Source: CAD feature listing. Evaluate the final solid. Frame: model axes, mm. A direction names the side the tool comes from. Round coordinates to 2 decimals unless told otherwise and drop trailing zeros. Loops run counter-clockwise (first coordinate to the right, second up) from the corner with the lowest first, then second, coordinate; pieces in that order, holes last. Notation, with made-up numbers: (20, 27.5) - (71, 27.5) arc R21 cw to (71, 37.5) - close; hole circle Ø7 at (1.5, 81). An arc over 180 degrees is marked (long way). One line per question, with ' | ' between items. Start each with the question number.
1. Pin query (flat end, axial travel): pin 1 (3 mm diameter, centred on x = -3, y = -6, fed in from -Z); pin 2 (3.5 mm diameter, centred on x = -1.5, y = -7, fed in from +Z); pin 3 (2 mm diameter, centred on x = 22, z = 9.5, fed in from +Y); pin 4 (6 mm diameter, centred on y = -6.5, z = 9, fed in from +X). Return the tip coordinate at first contact, or that it passes through.
2. Mould query, pull axis X, two halves, no side actions, for faces 4 (the cylindrical face through (14.75, -4.11, 32.57)), 5 (the flat face through (13, -12, 16)), 6 (the flat face through (0, -6, 8)). Classes: pulls with the +X half, pulls with the -X half, needs draft (parallel to the pull), parting line crosses it, or undercut.
3. Access query for faces 1 (the flat face through (7.5, -6, 26)), 2 (the flat face through (8, -6, 31)), 3 (the flat face through (13, 0, 16)). Directions: +Z, -Z, +X, -X, +Y, -Y. A direction counts if a zero-diameter tool reaches every point of the face in a straight line with its end or side. Return the directions, or none.
4. Cut plane B-B (x = 25.5). Return loops of the section in (y, z), then the cut area to 3 significant figures.
5. Cut plane A-A (x = -3). Return loops of the section in (y, z).
6. Cut plane C-C (z = 19.5). Return loops of the section in (x, y) (1 decimal).
7. Ray query, line 1 (Y direction, x = -3, z = 20); line 2 (Y direction, x = 15, z = 32.3) (3 decimals); line 3 (Z direction, x = 23, y = -11). Return the intervals inside material, ascending.
8. Cut plane D-D (x = 15). Return loops of the section in (y, z) (3 decimals).
```python
from build123d import *

# Parameters (mm, degrees)
F0_W     = 10
F0_H     = 4
F0_W_2   = 15
F0_H_2   = 9
F1_DEPTH = 12
F2_R     = 1.5875
F3_DEPTH = 10
F4_R     = 6.35
F4_R_2   = 1.905
F5_DEPTH = 3.175


with BuildPart() as f1:
    # F0 (on Front) → F1 (new body)
    with BuildSketch(Plane.XZ):
        Polygon((0, 16), (0, 0), (22.5, 0), (22.5, 4), (22.5, 16), align=None)
        with Locations((27.5, 2)):
            Rectangle(F0_W, F0_H)
        Polygon((-5, 16), (0, 16), (22.5, 16), (27.5, 16), (27.5, 22), (22.5, 22), (7.5, 22), (-5, 22), align=None)
        with Locations((15, 26.5)):
            Rectangle(F0_W_2, F0_H_2)
    extrude(amount=F1_DEPTH)

    # F2 (on face) → F3 (cut)
    with BuildSketch(Plane.XY.offset(22)):
        with Locations((-3, -6)):
            Circle(F2_R)
        with Locations((25.5, -6)):
            Circle(F2_R)
    extrude(amount=-F3_DEPTH, mode=Mode.SUBTRACT)

    # F4 (on face) → F5 (join)
    with BuildSketch(Plane.XY.offset(31)):
        with Locations((15, -6)):
            Circle(F4_R)
        with Locations((15, -6)):
            Circle(F4_R_2, mode=Mode.SUBTRACT)
    extrude(amount=F5_DEPTH)


solid = f1.part
```
Answers follow:
1) pin 1: passes through | pin 2: stops at z = 22 | pin 3: stops at y = 0 | pin 4: stops at x = 22.5
2) face 4: undercut | face 5: needs draft | face 6: pulls with the -X half
3) face 1: +Z, -X, +Y, -Y | face 2: +Z, -X | face 3: -Z, +X, -X, +Y
4) outline: (-12, 0) - (0, 0) - (0, 4) - (-12, 4) - close; (-12, 16) - (-7.59, 16) - (-7.59, 22) - (-12, 22) - close; (-4.41, 16) - (0, 16) - (0, 22) - (-4.41, 22) - close | area: 101 mm2
5) outline: (-12, 16) - (-7.59, 16) - (-7.59, 22) - (-12, 22) - close; (-4.41, 16) - (0, 16) - (0, 22) - (-4.41, 22) - close
6) outline: (-5, -12) - (27.5, -12) - (27.5, 0) - (-5, 0) - close; hole circle Ø3.2 at (-3, -6); hole circle Ø3.2 at (25.5, -6)
7) line 1: y = -12 to -7.59, -4.41 to 0 | line 2: y = -12.35 to -7.905, -4.095 to 0.35 | line 3: z = 0 to 4, 16 to 22
8) outline: (-12.35, 31) - (-12, 31) - (-12, 0) - (0, 0) - (0, 31) - (0.35, 31) - (0.35, 34.175) - (-4.095, 34.175) - (-4.095, 31) - (-7.905, 31) - (-7.905, 34.175) - (-12.35, 34.175) - close
